Autodesk Inventor part; units mm, degrees
ref_plane "YZ Plane" through (0, 0, 0) normal (1, 0, 0) x (0, 1, 0)
ref_plane "XZ Plane" through (0, 0, 0) normal (0, 1, 0) x (-1, 0, 0)
ref_plane "XY Plane" through (0, 0, 0) normal (0, 0, 1) x (1, 0, 0)
sketch "Sketch1" plane through (0, 0, 0) normal (0, 1, 0) x (-1, 0, 0)
  line L0 (3.5, 0) -> (-5.6696, 0) construction
  line L1 (0, -2.85) -> (3.5, -2.85)
  arc A0 (3.5, -2.85) -> (6.35, 0) centre (3.5, 0) ccw
  line L2 (0, 0) -> (0, -2.85)
  line L3 (0, 0) -> (6.35, 0)
  point P0 (-1.0848, 0)
  dimension "d0" = 2.85
  dimension "d1" = 3.5
revolve "Revolution1" add sketch "Sketch1" angle 360 about axis through (-3.5, 0, 0) along (1, 0, 0)
sketch "Sketch2" plane through (0, 0, 0) normal (0, 0, 1) x (1, 0, 0)
  arc A0 (-7.7327, 3.9972) -> (-7.7396, -4.0028) centre (-10.9, 0) ccw
  line L0 (0, -2.85) -> (0, 2.85)
  line L1 (-3.5, -2.4597) -> (-7.7396, -4.0028)
  line L2 (-3.5, 2.4567) -> (-7.7327, 3.9972)
  arc A1 (-3.5, 2.85) -> (-6.35, 0) centre (-3.5, 0) ccw
  line L3 (-3.5, 2.85) -> (0, 2.85)
  line L4 (0, 2.85) -> (0, -2.85)
  line L5 (0, -2.85) -> (-3.5, -2.85)
  arc A2 (-6.35, 0) -> (-3.5, -2.85) centre (-3.5, 0) ccw
  line L6 (-3.5, 2.4567) -> (-3.5, -2.4597)
  line L7 (-3.5, -2.85) -> (-3.5, 2.85)
  point P0 (0, 0)
  dimension "d3" = 10.2
  dimension "d4" = 10.9
  dimension "d7" = 8
  dimension "d12" = 110
  dimension "d13" = 110
extrude "Extrusion1" add sketch "Sketch2" along normal mid plane 2.9 contours L2 A1 A2 L1 A0 | L2 L6 L1 A2 A1
hole "Hole1" at (0, 0, 0) direction (-1, 0, 0) diameter 2.459 depth 6 tip angle 118
ref_plane "Work Plane1" through (-10.9, 0, 0) normal (1, 0, 0) x (0, 0, 1)
sketch "Sketch3" plane through (-10.9, 0, 0) normal (1, 0, 0) x (0, 0, 1)
  line L0 (-1.45, -5.1) -> (-1.45, 5.1)
  line L1 (-1.45, 5.1) -> (1.45, 5.1)
  line L2 (1.45, 5.1) -> (1.45, -5.1)
  line L3 (1.45, -5.1) -> (-1.45, -5.1)
  arc A0 (1.45, 2.8526) -> (-1.45, 2.8526) centre (0, 0) ccw
  line L4 (1.45, 0) -> (-1.45, 0)
  line L5 (-1.45, 2.8526) -> (-1.45, 0)
  line L6 (1.45, 0) -> (1.45, 2.8526)
  line L7 (-3.99, 0) -> (3.99, 0)
revolve "Revolution2" cut sketch "Sketch3" angle 360 about axis through (-10.9, 0, 0) along (0, 0, 1) contours L0 A0 L2 L4
sketch "Sketch4" plane through (0, 0, 1.45) normal (0, 0, 1) x (1, 0, 0)
  point P0 (0, 0)
  point P1 (-6.7959, 0)
hole "Hole2" at (-6.7959, 0, 1.45) direction (0, 0, -1) diameter 1 depth 0.5 tip angle 118
properties part number "500-103" material "Steel"
The listing builds one solid part. Answer for the finished solid, in the listing's coordinates (mm). A direction names the side the tool comes from. Give positions to 0.01 mm unless a question says otherwise; leave off trailing zeros. Order: outer loops, then holes, each group sorted by start corner. A loop starts at its lowest first (then second) coordinate and runs counter-clockwise, first axis right, second up. Notation, with made-up numbers: M 77.25,30.25 L 88.25,30.25 A24 ccw 88.25,54.25 Z; hole C -13,80.5 d3. An arc over 180 degrees is marked long. Put each result on its own line as item: value. Start each with the question number.
Item 1: Flat-ended cylindrical pins translate along their axes: P1, Ø6, axis at x = -14, y = -3, coming from the +Z side; P2, Ø3, axis at y = -2, z = 1, coming from the -X side. Find the tip coordinate at first contact, or state that the pin passes through.
Item 2: Find the intervals of material crossed by line 1 along Z through (x, y) = (-1.65, 0); line 2 along X through (y, z) = (0, 1.1), in increasing order.
Item 3: For a pull along X with two mould halves and no side action, classify faces 1 (the face through (-7.29, 0.07, 1.2)), 2 (the face through (-8, 2, 1.45)), 3 (the face through (-16, 0, 0)) as +X half, -X half, draft (parallel to the pull), parting line (faces both ways), or undercut.
Item 4: The part is cut by section D-D, the plane y = -1.5. Determine the outline of the cut face in (x, z), and give its area (3 significant figures).
Item 5: The part is cut by section C-C, the plane x = -3. Determine the outline of the cut face in (y, z).
Item 6: The part is cut by section A-A, the plane y = 2. Determine the outline of the cut face in (x, z).
Item 7: The part is cut by section B-B, the plane x = -11.75. Determine the outline of the cut face in (y, z), and give its area (3 significant figures).
Item 8: Which of the six approach directions +Z, -Z, +X, -X, +Y, -Y give full straight-line access (tool end or side, diameter ignored) to faces 4 (the face through (-1.774, 1.734, 2.262)), 5 (the face through (-6.849, 0.069, 0.702))?
Answer key:
1. P1: stops at z = 1.45
1. P2: stops at x = -15.98
2. line 1: z = -2.85 to -1.23, 1.23 to 2.85
2. line 2: x = -16 to -13.9, -7.9 to -7.3, -6.3 to -6.08
3. face 1: undercut
3. face 2: draft
3. face 3: parting line
4. outline: M -15.77,-1.45 L -13.33,-1.45 A2.83 cw -13.33,1.45 L -15.77,1.45 Z; M -8.47,-1.45 L -5.44,-1.45 A2.42 ccw -3.5,-2.42 L 0,-2.42 L 0,2.42 L -3.5,2.42 A2.42 ccw -5.44,1.45 L -8.47,1.45 A2.83 cw Z
4. area: 39.6 mm²
5. outline: C 0,0 d5.7; hole C 0,0 d2.46
6. outline: M -15.59,-1.45 L -12.93,-1.45 A2.5 cw -12.93,1.45 L -15.59,1.45 Z; M -8.87,-1.45 L -4.92,-1.45 A2.03 ccw -3.5,-2.03 L 0,-2.03 L 0,2.03 L -3.5,2.03 A2.03 ccw -4.92,1.45 L -8.87,1.45 A2.5 cw Z
7. outline: M -5.03,-1.45 L -2.72,-1.45 A3.09 cw -2.72,1.45 L -5.03,1.45 Z; M 2.72,-1.45 L 5.03,-1.45 L 5.03,1.45 L 2.72,1.45 A3.09 cw Z
7. area: 12.0 mm²
8. face 4: +X
8. face 5: +Z
